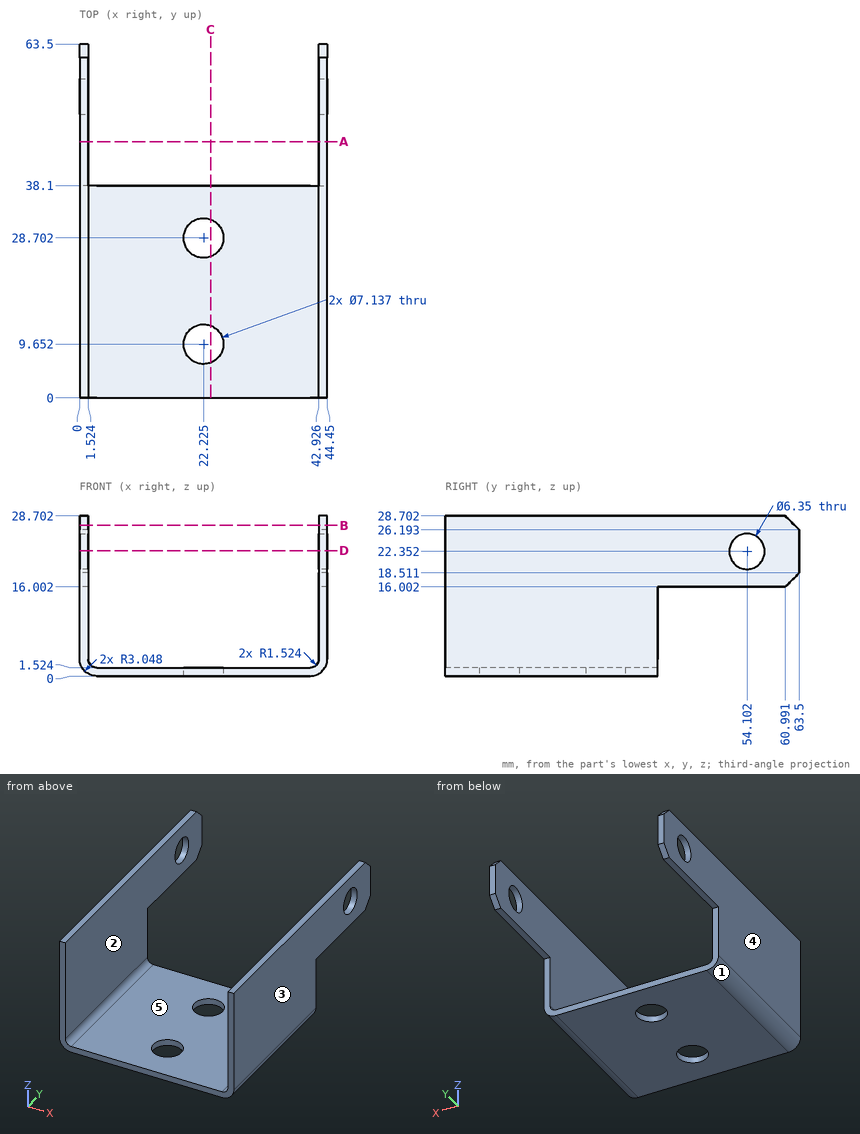
Verification items for this drawing (mm, ordinates from the low corner). A direction names the side the tool comes from. Give positions to 0.01 mm unless a question says otherwise; leave off trailing zeros. Loops run counter-clockwise (first coordinate to the right, second up) from the corner with the lowest first, then second, coordinate; pieces in that order, holes last.
1. Cross-section at C-C on x = 23.5. Record the cut outline in (y, z) (1 decimal).
Derived:
outline: (0, 0) - (6.3, 0) - (6.3, 1.5) - (0, 1.5) - close; (13, 0) - (25.4, 0) - (25.4, 1.5) - (13, 1.5) - close; (32, 0) - (38.1, 0) - (38.1, 1.5) - (32, 1.5) - close
2. Go/stop test with flat-tipped pins: P1, Ø8, axis at x = 22.225, y = 9.652, coming from the +Z side; P2, Ø0.8, axis at x = 1, y = 44, coming from the -Z side. Record where each tip stops, or that it passes through.
Derived:
P1: stops at z = 1.52
P2: stops at z = 16
3. Cross-section at D-D on z = 22.5. Record the cut outline in (x, y), and give its area (3 significant figures).
Derived:
outline: (0, 0) - (1.52, 0) - (1.52, 50.93) - (0, 50.93) - close; (0, 57.27) - (1.52, 57.27) - (1.52, 63.5) - (0, 63.5) - close; (42.93, 0) - (44.45, 0) - (44.45, 50.93) - (42.93, 50.93) - close; (42.93, 57.27) - (44.45, 57.27) - (44.45, 63.5) - (42.93, 63.5) - close
area: 174 mm2
4. Tool access check on the marked faces 4 and 5. Record the directions out of +Z, -Z, +X, -X, +Y, -Y that give a thin tool (end or side, any length) a straight path to the whole face; none if there is none.
Derived:
face 4: +Z, -Z, -X, +Y, -Y
face 5: +Z, +Y, -Y
5. Cross-section at A-A on y = 46. Record the cut outline in (x, z).
Derived:
outline: (0, 16) - (1.52, 16) - (1.52, 28.7) - (0, 28.7) - close; (42.93, 16) - (44.45, 16) - (44.45, 28.7) - (42.93, 28.7) - close
6. Material ranges on probe 1 along X at (y, z) = (12.5, 19.25); probe 2 along Z at (x, y) = (17.5, 11); probe 3 along X at (y, z) = (15, 2.75) (1 decimal), recorded low to high.
Derived:
probe 1: x = 0 to 1.52, 42.93 to 44.45
probe 2: z = 0 to 1.52
probe 3: x = 0 to 1.6, 42.9 to 44.4
7. Release check for a two-part mould opening along X. For the marked faces 1, 2 and 3 record: +X half, -X half, draft (parallel to the pull), parting line (faces both ways), or undercut.
Derived:
face 1: -X half
face 2: undercut
face 3: +X half
8. Cross-section at B-B on z = 27. Record the cut outline in (x, y), and give its area (3 significant figures).
Derived:
outline: (0, 0) - (1.52, 0) - (1.52, 62.69) - (0, 62.69) - close; (42.93, 0) - (44.45, 0) - (44.45, 62.69) - (42.93, 62.69) - close
area: 191 mm2
